Here's how the part is built. I have some questions about the finished solid (model axes, mm). Face numbers are marked on the shaded views. Give positions to 0.01 mm unless a question says otherwise; leave off trailing zeros. Loops run counter-clockwise (first coordinate to the right, second up) from the corner with the lowest first, then second, coordinate; pieces in that order, holes last. Notation, with made-up numbers: (73, 0.5) - (84, 0.5) arc R22 cw to (84, 33.5) - close; hole circle Ø2 at (22, -4.75). An arc over 180 degrees is marked (long way). Return JSON: item names as keys, results as strings. Group by question number.
(1) If we section it at A-A (z = 0): Please give me the cut outline in (x, y).
(2) If we section it at B-B (y = 2.45): Please give me the cut outline in (x, z).
(3) If we section it at C-C (z = 20): Please give me the cut outline in (x, y), then the cut area to 3 significant figures.
(4) For P1, Ø8, axis at x = 20, z = -20, coming from the +Y side; P2, Ø4.5, axis at x = 20, z = 20, coming from the -Y side, each with a flat end and sliding along its axis, tell me the tip position at first contact or that it passes through.
(5) I need wall thicknesses on probe 1 along Z at (x, y) = (20, 1.25); probe 2 along X at (y, z) = (4.3, -22); probe 3 along Z at (x, y) = (-19, 3.15). Which ranges of each line are inside material? Lowest first, please. Write a range as [from, to].
(6) If we mould it in two halves opening along X, with no side actions, what happens to the marked faces 1, 2, 3 and 4? For each: released by +X, released by -X, zero draft, split by the parting line, or undercut.
(7) If we section it at D-D (x = 20): Please give me the cut outline in (y, z).
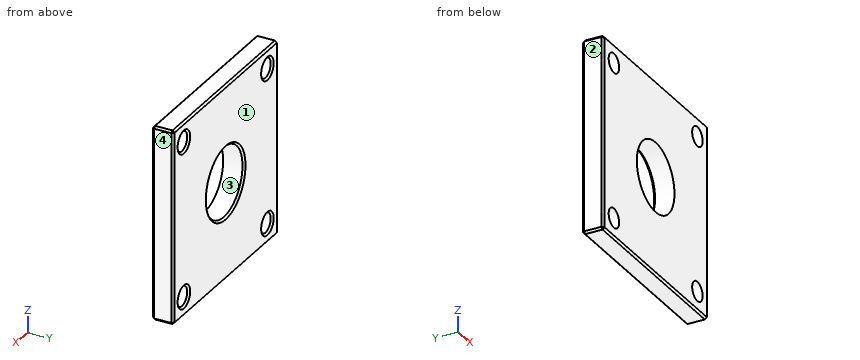
```python
from build123d import *

# Parameters (mm, degrees)
F0_W     = 50
F0_H     = 50
F1_DEPTH = 5.5
F2_R     = 9
F3_DEPTH = 25
F4_R     = 2.5
F5_DEPTH = 25
F6_SIZE  = 0.5


with BuildPart() as f1:
    # F0 (on Front) → F1 (new body)
    with BuildSketch(Plane.XZ):
        Rectangle(F0_W, F0_H)
    extrude(amount=-F1_DEPTH)

    # F2 (on face) → F3 (cut)
    with BuildSketch(Plane.XZ):
        Circle(F2_R)
    extrude(amount=-F3_DEPTH, mode=Mode.SUBTRACT)

    # F4 (on face) → F5 (cut)
    with BuildSketch(Plane.XZ):
        with Locations((-20, -20)):
            Circle(F4_R)
        with Locations((20, -20)):
            Circle(F4_R)
        with Locations((-20, 20)):
            Circle(F4_R)
        with Locations((20, 20)):
            Circle(F4_R)
    extrude(amount=-F5_DEPTH, mode=Mode.SUBTRACT)

    # F6
    f6_edges = [f1.edges().sort_by_distance(p)[0] for p in [
        (0, 0, -25),
        (-25, 0, 0),
        (0, 0, 25),
        (25, 0, 0),
        (25, 2.75, -25),
        (-25, 2.75, -25),
        (-25, 2.75, 25),
        (25, 2.75, 25),
        (0, 5.5, 25),
        (25, 5.5, 0),
        (0, 5.5, -25),
        (-25, 5.5, 0),
        (-22.5, 5.5, -20),
        (17.5, 5.5, -20),
        (-22.5, 5.5, 20),
        (-9, 5.5, 0),
        (17.5, 5.5, 20),
    ]]
    chamfer(f6_edges, length=F6_SIZE)


solid = f1.part
```
Values:
{
 "1": {"outline": "(-25, 0.5) - (-24.5, 0) - (-9, 0) - (-9, 5) - (-9.5, 5.5) - (-24.5, 5.5) - (-25, 5) - close; (9, 0) - (24.5, 0) - (25, 0.5) - (25, 5) - (24.5, 5.5) - (9.5, 5.5) - (9, 5) - close"},
 "2": {"outline": "(-25, -24.5) - (-24.5, -25) - (24.5, -25) - (25, -24.5) - (25, 24.5) - (24.5, 25) - (-24.5, 25) - (-25, 24.5) - close; hole circle Ø5 at (-20, -20); hole circle Ø5 at (-20, 20); hole circle Ø18 at (0, 0); hole circle Ø5 at (20, -20); hole circle Ø5 at (20, 20)"},
 "3": {"outline": "(-25, 0.5) - (-24.5, 0) - (-22.5, 0) - (-22.5, 5) - (-23, 5.5) - (-24.5, 5.5) - (-25, 5) - close; (-17.5, 0) - (17.5, 0) - (17.5, 5) - (17, 5.5) - (-17, 5.5) - (-17.5, 5) - close; (22.5, 0) - (24.5, 0) - (25, 0.5) - (25, 5) - (24.5, 5.5) - (23, 5.5) - (22.5, 5) - close", "area": "219 mm2"},
 "4": {"P1": "y = 5.5", "P2": "through"},
 "5": {"probe 1": "[-25, -22.5], [-17.5, 17.5], [22.5, 25]", "probe 2": "[-25, -21.5], [-18.5, 18.5], [21.5, 25]", "probe 3": "[-25, -22.29], [-17.71, 17.71], [22.29, 25]"},
 "6": {"face 1": "zero draft", "face 2": "released by -X", "face 3": "undercut", "face 4": "released by +X"},
 "7": {"outline": "(0, -24.5) - (0.5, -25) - (5, -25) - (5.5, -24.5) - (5.5, -23) - (5, -22.5) - (0, -22.5) - close; (0, -17.5) - (5, -17.5) - (5.5, -17) - (5.5, 17) - (5, 17.5) - (0, 17.5) - close; (0, 22.5) - (5, 22.5) - (5.5, 23) - (5.5, 24.5) - (5, 25) - (0.5, 25) - (0, 24.5) - close"}
}
